CAD build for the part. Positions are in the model's coordinates, mm. A direction names the side the tool comes from. Coordinates: 2 decimals unless noted, no trailing zeros. Write each loop counter-clockwise with the first axis right and the second up, starting at its lowest first coordinate (ties: lowest second). Pieces come first, ordered by that corner, then holes. Notation, with made-up numbers: (68.25, -40) -> (115.25, -40) arc R21 ccw to (115.25, -5) -> close; hole circle Ø6 at (55, 37). An arc over 180 degrees is marked (long way). Answer as CSV lines item,"result".
```python
from build123d import *

# Parameters (mm, degrees)
BOSS_EXTRUDE1_DEPTH      = 6
BOSS_EXTRUDE1_DEPTH_BACK = 6
SKETCH2_W                = 156
SKETCH2_H                = 8
CUT_EXTRUDE1_DEPTH       = 160
SKETCH4_W                = 38
SKETCH4_H                = 12
CUT_EXTRUDE2_DEPTH       = 12
CUT_EXTRUDE3_DEPTH       = 114.296072306
CUT_EXTRUDE3_DEPTH_BACK  = 114.296072306
SKETCH6_R                = 1.5
CUT_EXTRUDE4_REACH       = 180.986
SKETCH7_R                = 1.75
SKETCH8_W                = 12
SKETCH8_H                = 16
CUT_EXTRUDE5_DEPTH       = 2
SKETCH9_W                = 12
SKETCH9_H                = 28
CUT_EXTRUDE6_DEPTH       = 1
CUT_EXTRUDE7_DEPTH       = 2
BOSS_EXTRUDE2_DEPTH      = 10


with BuildPart() as part:
    # Sketch1 → Boss-Extrude1 (new, two sides: drawn at the far end of the back side and taken through both)
    with BuildSketch(Plane(origin=(0, 0, 0), x_dir=(1, 0, 0), z_dir=(0, 1, 0)).offset(-BOSS_EXTRUDE1_DEPTH_BACK)):
        Polygon((80, 15), (80, -15), (40, -15), (40, -65), (80, -72), (80, -80), (74, -80), (0, -67.05), (-74, -80), (-80, -80), (-80, -72), (-40, -65), (-40, -15), (-80, -15), (-80, 15), (-40, 15), (-40, 65), (-80, 72), (-80, 80), (-74, 80), (0, 67.05), (74, 80), (80, 80), (80, 72), (40, 65), (40, 15), align=None)
    extrude(amount=BOSS_EXTRUDE1_DEPTH + BOSS_EXTRUDE1_DEPTH_BACK)

    # Sketch2 → Cut-Extrude1 (cut)
    with BuildSketch(Plane.XY.offset(80)):
        Rectangle(SKETCH2_W, SKETCH2_H)
    extrude(amount=-CUT_EXTRUDE1_DEPTH, mode=Mode.SUBTRACT)

    # Sketch4 → Cut-Extrude2 (cut)
    with BuildSketch(Plane(origin=(0, 6, 0), x_dir=(1, 0, 0), z_dir=(0, 1, 0))):
        with Locations((-59, 0)):
            Rectangle(SKETCH4_W, SKETCH4_H)
        with Locations((59, 0)):
            Rectangle(SKETCH4_W, SKETCH4_H)
    extrude(amount=-CUT_EXTRUDE2_DEPTH, mode=Mode.SUBTRACT)

    # Sketch6 → Cut-Extrude3 (cut, two sides: drawn at the far end of the back side and taken through both)
    with BuildSketch(Plane(origin=(0, 0, 0), x_dir=(0, 0, -1), z_dir=(1, 0, 0)).offset(-CUT_EXTRUDE3_DEPTH_BACK)):
        with Locations((-76, 0)):
            Circle(SKETCH6_R)
        with Locations((76, 0)):
            Circle(SKETCH6_R)
    extrude(amount=CUT_EXTRUDE3_DEPTH + CUT_EXTRUDE3_DEPTH_BACK, mode=Mode.SUBTRACT)

    # Cut-Extrude4: up to this face of the body (flat: up to its plane)
    cut_extrude4_end = Plane(part.part.faces().sort_by_distance((-80, 0, 0))[0])
    # Sketch7 → Cut-Extrude4 (cut, up to the picked face)
    with BuildSketch(Plane(origin=(80, 0, 0), x_dir=(0, 0, -1), z_dir=(1, 0, 0)), mode=Mode.PRIVATE) as cut_extrude4_sk1:
        Circle(SKETCH7_R)
    cut_extrude4_tool1 = split(extrude(cut_extrude4_sk1.sketch, amount=-CUT_EXTRUDE4_REACH, mode=Mode.PRIVATE), bisect_by=cut_extrude4_end, keep=Keep.BOTH, mode=Mode.PRIVATE)
    add(cut_extrude4_tool1.solids().sort_by(Axis((80, 0, 0), (-1, 0, 0)))[0], mode=Mode.SUBTRACT)

    # Sketch8 → Cut-Extrude5 (cut)
    with BuildSketch(Plane(origin=(0, 6, 0), x_dir=(1, 0, 0), z_dir=(0, 1, 0))):
        with Locations((72, 0)):
            Rectangle(SKETCH8_W, SKETCH8_H)
        with Locations((-72, 0)):
            Rectangle(SKETCH8_W, SKETCH8_H)
    extrude(amount=-CUT_EXTRUDE5_DEPTH, mode=Mode.SUBTRACT)

    # Sketch9 → Cut-Extrude6 (cut)
    with BuildSketch(Plane(origin=(0, -4, 0), x_dir=(1, 0, 0), z_dir=(0, 1, 0))):
        with Locations((72, 0)):
            Rectangle(SKETCH9_W, SKETCH9_H)
        with Locations((-72, 0)):
            Rectangle(SKETCH9_W, SKETCH9_H)
    extrude(amount=-CUT_EXTRUDE6_DEPTH, mode=Mode.SUBTRACT)

    # Sketch11 → Cut-Extrude7 (cut)
    with BuildSketch(Plane(origin=(0, 6, 0), x_dir=(1, 0, 0), z_dir=(0, 1, 0))):
        Polygon((-40, -74.05), (-40, 74.05), (0, 67.05), (40, 74.05), (40, -74.05), (0, -67.05), align=None)
    extrude(amount=-CUT_EXTRUDE7_DEPTH, mode=Mode.SUBTRACT)

    # Sketch12 → Boss-Extrude2 (add)
    with BuildSketch(Plane(origin=(0, -4, 0), x_dir=(1, 0, 0), z_dir=(0, 1, 0))):
        Polygon((-40, 74.05), (-40, -74.05), (0, -67.05), (40, -74.05), (40, 74.05), (0, 67.05), align=None)
        Polygon((0, 65.01960595), (38, 71.66960595), (38, -71.66960595), (0, -65.01960595), (-38, -71.66960595), (-38, 71.66960595), align=None, mode=Mode.SUBTRACT)
    extrude(amount=BOSS_EXTRUDE2_DEPTH)


solid = part.part
```
Item 1: Two-plate mould, pull along X, no slides. Class faces 1 (the flat face through (-80, -1.4, -75.1)), 2 (the flat face through (61.4, -4.5, -15)), 3 (the flat face through (-78, -2, 76)), 4 (the flat face through (80, -3, 0)): pulls with the +X half, pulls with the -X half, needs draft (parallel to the pull), parting line crosses it, or undercut.
Answer below:
face 1,"pulls with the -X half"
face 2,"needs draft"
face 3,"undercut"
face 4,"pulls with the +X half"
Item 2: Flat gauge pins, fed straight in: pin 1 (1.5 mm diameter, centred on x = -5, y = 0, fed in from +Z); pin 2 (8 mm diameter, centred on x = 28.5, z = -9.5, fed in from +Y); pin 3 (3 mm diameter, centred on x = -1.5, y = -1.5, fed in from +Z) (3 decimals). Where does each tip first touch, or does it go through?
Answer below:
pin 1,"stops at z = 68.06"
pin 2,"stops at y = -4"
pin 3,"stops at z = 67.575"
Item 3: 3-axis set-ups, long thin cutter, end or side, ignore diameter. For faces 5 (the flat face through (-28.26, -0.084, -71.995)), 6 (the flat face through (-64.724, -5.417, 69.327)), 7 (the flat face through (38, 1, -1)): which of +Z, -Z, +X, -X, +Y, -Y reach the whole face in a straight line?
Answer below:
face 5,"-Z, +Y, -Y"
face 6,"-X, +Y, -Y"
face 7,"+Y"
Item 4: Saw through at B-B on x = -57. State how many separate pieces and enclosed holes the cut face has, and give its area (3 significant figures).
Answer below:
separate pieces,"8"
enclosed holes,"0"
area,"144 mm2"
Item 5: Wall check: line 1 (X direction, y = 2.5, z = 4); line 2 (X direction, y = -3.5, z = 57.5); line 3 (Y direction, x = -79, z = 76). Give the ranges that are in metal, low to high. Write a range as from..to.
Answer below:
line 1,"x = -80..-78, -40..-38, 38..40, 78..80"
line 2,"x = -40..-38, 38..40"
line 3,"y = -6..-1.5, 1.5..6"
Item 6: Saw through at C-C on x = -29.5. Give the cut face in (y, z), and give its area (3 significant figures).
Answer below:
outline,"(-6, -72.21) -> (6, -72.21) -> (6, -70.18) -> (-4, -70.18) -> (-4, 70.18) -> (6, 70.18) -> (6, 72.21) -> (-6, 72.21) -> close"
area,"329 mm2"
Item 7: Saw through at A-A on z = 21. Give the cut face in (x, y), and give its area (3 significant figures).
Answer below:
outline,"(-40, -6) -> (40, -6) -> (40, 6) -> (38, 6) -> (38, -4) -> (-38, -4) -> (-38, 6) -> (-40, 6) -> close"
area,"200 mm2"
